The model under review builds one solid part; all positions refer to its coordinate system, in mm. Face numbers are marked on the shaded views. Round coordinates to 2 decimals unless told otherwise and drop trailing zeros. Write each loop counter-clockwise with the first axis right and the second up, starting at its lowest first coordinate (ties: lowest second). Pieces come first, ordered by that corner, then holes. Notation, with made-up numbers: (-29.75, 47.25) -> (-11.75, 47.25) arc R19 ccw to (-11.75, 77.25) -> close; hole circle Ø1 at (59, 33). An arc over 180 degrees is marked (long way). Answer as a JSON object with one key per item and string values. Group by question number.
1) Mouldability with a two-part tool opening along Y and no side actions: class the marked faces 1, 2 and 3 as pulls with the +Y half, pulls with the -Y half, needs draft (parallel to the pull), parting line crosses it, or undercut.
2) To check wall thickness, follow probe 1 along Y at (x, z) = (0, 24); probe 2 along Y at (x, z) = (-27.5, 67); probe 3 along Z at (x, y) = (-37, -2.5). State the ranges of each line that lie inside material, in increasing order. Write a range as [from, to].
3) We need section B-B, the plane z = 18. Write out the cut boundary in (x, y).
4) Insertion check: pin 1 Ø10 at (x, z) = (4, 4) entering from -Y; pin 2 Ø5 at (x, y) = (5, 4) entering from +Z; pin 3 Ø5 at (x, z) = (40.5, 56.5) entering from +Y. Each pin has a flat end and moves straight along its axis. Give the tip position at first contact, or say it passes through.
from build123d import *

# Parameters (mm, degrees)
F0_R      = 51.7494214311
F1_DEPTH  = 76.2
F2_T      = -5.08
F1_FACE_R = 51.7494214311
F3_DEPTH  = 5.08
F4_R      = 2.53999
F5_R      = 5.08
F6_R      = 5.07999


# Not quite as in the source:
# - a fillet or chamfer is up to 0.001 mm smaller than in the source, because OpenCascade refuses the exact size


with BuildPart() as f1:
    # F0 (on Top) → F1 (new body)
    with BuildSketch(Plane.XY):
        Circle(F0_R)
    extrude(amount=F1_DEPTH)

    # F2
    f2_openings = [f1.faces().sort_by_distance(p)[0] for p in [
        (0, 0, 76.2),
    ]]
    offset(amount=F2_T, openings=f2_openings)

    # F0 (on Top) + F1_face (on face) → F3 (join)
    with BuildSketch(Plane.XY):
        Circle(F0_R)
    with BuildSketch(Plane(origin=(0, 0, 0), x_dir=(1, 0, 0), z_dir=(0, 0, -1))):
        Circle(F1_FACE_R)
    extrude(amount=-F3_DEPTH, dir=(0, 0, 1))

    # F4 (radius 2.54 in the source; OpenCascade refuses exactly that, so slightly less here)
    f4_edges = [f1.edges().sort_by_distance(p)[0] for p in [
        (-51.749421, 0, 76.2),
        (-46.669421, 0, 76.2),
    ]]
    fillet(f4_edges, radius=F4_R)

    # F5
    f5_edges = [f1.edges().sort_by_distance(p)[0] for p in [
        (-46.669421, 0, 5.08),
    ]]
    fillet(f5_edges, radius=F5_R)

    # F6 (radius 5.08 in the source; OpenCascade refuses exactly that, so slightly less here)
    f6_edges = [f1.edges().sort_by_distance(p)[0] for p in [
        (-51.749421, 0, -5.08),
    ]]
    fillet(f6_edges, radius=F6_R)


solid = f1.part
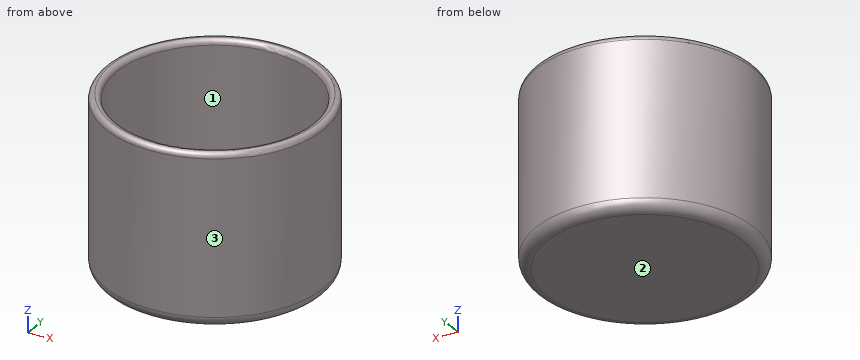
Here are the results:
{
 "1": {"face 1": "undercut", "face 2": "needs draft", "face 3": "parting line crosses it"},
 "2": {"probe 1": "y = [-51.75, -46.67], [46.67, 51.75]", "probe 2": "y = [-43.84, -37.71], [37.71, 43.84]", "probe 3": "z = [-5.08, 5.08]"},
 "3": {"outline": "circle Ø103.5 at (0, 0); hole circle Ø93.34 at (0, 0)"},
 "4": {"pin 1": "stops at y = -51.75", "pin 2": "stops at z = 5.08", "pin 3": "stops at y = 35.13"}
}
